Autodesk Inventor part; units mm, degrees
ref_plane "YZ Plane" through (0, 0, 0) normal (1, 0, 0) x (0, 1, 0)
ref_plane "XZ Plane" through (0, 0, 0) normal (0, 1, 0) x (-1, 0, 0)
ref_plane "XY Plane" through (0, 0, 0) normal (0, 0, 1) x (1, 0, 0)
sketch "Skizze1" plane through (0, 0, 0) normal (0, 0, 1) x (1, 0, 0)
  line L0 (0, 0) -> (200, 0)
  line L1 (200, 0) -> (200, 3)
  line L2 (200, 3) -> (0, 3)
  line L3 (0, 3) -> (0, 0)
  dimension "d0" = 200
  dimension "d1" = 3
extrude "Extrusion1" add sketch "Skizze1" along normal blind 3
sketch "Skizze2" plane through (200, 0, 0) normal (1, 0, 0) x (0, 0, -1)
  point P0 (0, 0)
sketch "Skizze3" plane through (0, 0, 0) normal (0, -1, 0) x (1, 0, 0)
  line L0 (0, 0) -> (200, 0)
  line L1 (200, 0) -> (53.164, 0)
  dimension "d4" = 146.836
sketch "Skizze4" plane through (10, 0, 0) normal (-1, 0, 0) x (0, 0, 1)
  line L0 (0, 3) -> (3, 3)
  line L1 (0, 0) -> (3, 3)
  line L2 (3, 3) -> (0, 3)
  line L3 (0, 3) -> (3, 0)
  line L4 (-1.5, -1.5) -> (4.5, -1.5)
  line L5 (4.5, -1.5) -> (4.5, 4.5)
  line L6 (4.5, 4.5) -> (-1.5, 4.5)
  line L7 (-1.5, 4.5) -> (-1.5, -1.5)
  line L8 (-1.5, -1.5) -> (4.5, 4.5) construction
  line L9 (4.5, -1.5) -> (-1.5, 4.5) construction
  point P0 (1.5, 1.5)
  dimension "d14" = 6
  dimension "d15" = 6
extrude "Extrusion2" add sketch "Skizze4" along normal blind 10 contours L0 L1 L3 | L7 L6 L5 L4
chamfer "Fase1" distance 2.99 distance2 10 1 edges at (0, 1.5, -1.5) measured on face at (0, 2.5, 0.5)
chamfer "Fase2" distance 2.99 distance2 10 1 edges at (0, 1.5, 4.5) measured on face at (0, 2.5, 2.493)
chamfer "Fase3" distance 2.99 distance2 10 1 edges at (0, -1.5, 1.5) measured on face at (0, 0.5, 1.5035)
chamfer "Fase4" distance 2.99 distance2 10 1 edges at (0, 4.5, 1.5) measured on face at (0, 3.4965, 1.4965)
sketch "Skizze9" plane through (10, 0, 0) normal (0, -1, 0) x (1, 0, 0)
  line L0 (0, 3) -> (190, 3)
  line L1 (40.0497, 3) -> (40.0497, 0)
  line L2 (0, 0) -> (190, 0)
  point P0 (-10, 0)
sketch "Skizze10" plane through (0, 0, 0) normal (0, 0, -1) x (-1, 0, 0)
  line L0 (-200, 3) -> (-10, 3)
  line L1 (-51.2532, 3) -> (-50.0501, 0)
  line L2 (-10, 0) -> (-200, 0)
  point P0 (0, 0)
properties part number "blueStick"
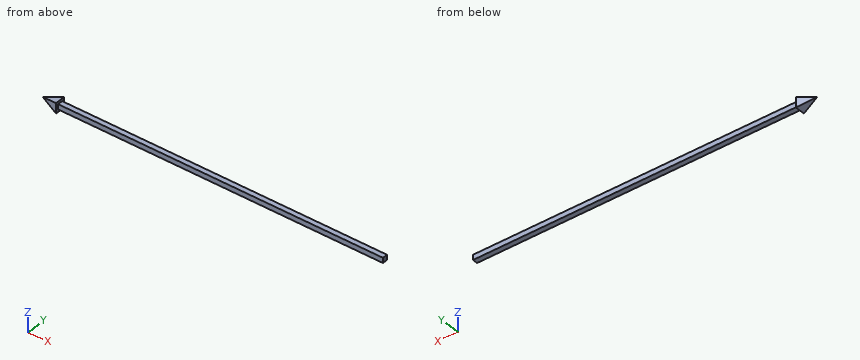
CAD build for the part. Positions are in the model's coordinates, mm. Coordinates: 2 decimals unless noted, no trailing zeros. Order: outer loops, then holes, each group sorted by start corner. A loop starts at its lowest first (then second) coordinate and runs counter-clockwise, first axis right, second up. Notation, with made-up numbers: (61.5, -11.75) - (90.5, -11.75) arc R16 ccw to (90.5, 16.25) - close; hole circle Ø8 at (83.5, 36). An arc over 180 degrees is marked (long way). Use a Markdown table: item, result. Add a question column.
(1) Flat gauge pins, fed straight in: pin 1 (1.5 mm diameter, centred on x = 145, z = 2, fed in from -Y); pin 2 (1.5 mm diameter, centred on x = 102.5, y = 2, fed in from -Z); pin 3 (1.5 mm diameter, centred on y = 0.5, z = -1, fed in from +X). Where does each tip first touch, or does it go through?
(2) Saw through at A-A (x = 71). Give the cut face in (y, z).
(3) Drill centre line: line 1 along Y through (x, z) = (185, 0.25). Where is it in solid material? Low to high. Write a range as [from, to].
Solved:
| question | item | result |
|---|---|---|
| 1 | pin 1 | stops at y = 0 |
| 1 | pin 2 | stops at z = 0 |
| 1 | pin 3 | stops at x = 10 |
| 2 | outline | (0, 0) - (3, 0) - (3, 3) - (0, 3) - close |
| 3 | line 1 | y = [0, 3] |
